Geometry check sheet. Reference: the model listing, model coordinates, mm. A direction names the side the tool comes from. Give positions to 0.01 mm unless a question says otherwise; leave off trailing zeros. Write each loop counter-clockwise with the first axis right and the second up, starting at its lowest first coordinate (ties: lowest second). Pieces come first, ordered by that corner, then holes.
(1) Cross-section at D-D (x = -11.5). Record the boundary of the cut face in (y, z) (3 decimals), and give its area (3 significant figures).
(2) Cross-section at C-C (z = 1.1). Count the separate pieces of the cut face and the enclosed holes in it, and give its area (3 significant figures).
(3) Thickness scan on line 1 along Y through (x, z) = (0, 2.65); line 2 along Y through (x, z) = (0, 3.95); line 3 along X through (y, z) = (-5.5, 0.45). Record the ranges inside material, lowest first.
(4) Tool access check on faces 3 (the flat face through (-11, -6.645, 2)), 4 (the cylindrical face through (-0.88, -3.94, 4.24)). Record the directions out of +Z, -Z, +X, -X, +Y, -Y that give a thin tool (end or side, any length) a straight path to the whole face; none if there is none.
(5) Mould release check, pull along X, two halves, no side actions. Record for faces 1 (the flat face through (6.645, -11, 2)), 2 (the flat face through (-5, 5, 0)): +X half, -X half, draft (parallel to the pull), parting line (faces both ways), or undercut.
(6) Depth check by flat-ended pin: P1, Ø1.4, axis at x = 12, y = -2.5, coming from the -Z side (3 decimals); P2, Ø0.7, axis at x = -11, z = 1, coming from the -Y side; P3, Ø1.2, axis at y = -10.5, z = 1, coming from the +X side. Enter the tip coordinate at first touch or a pass-through.
```python
from build123d import *

# Parameters (mm, degrees)
SKETCH1_R               = 15
BOSS_EXTRUDE1_DEPTH     = 5
CUT_EXTRUDE1_DEPTH      = 3.125
BOSS_EXTRUDE4_START     = 3.125
BOSS_EXTRUDE4_DEPTH     = 3.125
CIRPATTERN1_COUNT       = 4
SKETCH4_R               = 6
CUT_EXTRUDE2_DEPTH      = 3.5
FILLET1_R               = 0.25
CUT_EXTRUDE3_DEPTH      = 22.794494718
CUT_EXTRUDE3_DEPTH_BACK = 22.794494718
SKETCH5_R               = 4.0375
FILLET2_R               = 0.5


with BuildPart() as part:
    # Sketch1 → Boss-Extrude1 (new body)
    with BuildSketch(Plane.XY):
        Circle(SKETCH1_R)
    extrude(amount=BOSS_EXTRUDE1_DEPTH)

    # Sketch1_5 → Cut-Extrude1 (cut)
    with BuildSketch(Plane.XY):
        with BuildLine():
            ThreePointArc((-2.469224322, 13.9075), (-4.680749466, 13.326897968), (-6.769624128, 12.397088939))
            Line((-6.769624128, 12.397088939), (-6.769624128, 8.9075))
            Line((-6.769624128, 8.9075), (6.769624128, 8.9075))
            Line((6.769624128, 8.9075), (6.769624128, 12.397088939))
            ThreePointArc((6.769624128, 12.397088939), (4.680749466, 13.326897968), (2.469224322, 13.9075))
            Line((2.469224322, 13.9075), (-2.469224322, 13.9075))
        make_face()
    cut_extrude1 = extrude(amount=CUT_EXTRUDE1_DEPTH, mode=Mode.SUBTRACT)

    # Sketch7 → Boss-Extrude4 (add)
    with BuildSketch(Plane(origin=(0, 0, 3.125), x_dir=(-1, 0, 0), z_dir=(0, 0, -1)).offset(BOSS_EXTRUDE4_START)):
        with BuildLine():
            ThreePointArc((-2.469224322, 13.9075), (-4.680749466, 13.326897968), (-6.769624128, 12.397088939))
            Line((-6.769624128, 12.397088939), (-6.769624128, 8.9075))
            Line((-6.769624128, 8.9075), (6.769624128, 8.9075))
            Line((6.769624128, 8.9075), (6.769624128, 12.397088939))
            ThreePointArc((6.769624128, 12.397088939), (4.680749466, 13.326897968), (2.469224322, 13.9075))
            Line((2.469224322, 13.9075), (-2.469224322, 13.9075))
        make_face()
        with BuildLine():
            ThreePointArc((-2.45818912, 13.7825), (-4.609561284, 13.219377624), (-6.644624128, 12.322701416))
            Line((-6.644624128, 12.322701416), (-6.644624128, 9.0325))
            Line((-6.644624128, 9.0325), (6.644624128, 9.0325))
            Line((6.644624128, 9.0325), (6.644624128, 12.322701416))
            ThreePointArc((6.644624128, 12.322701416), (4.609561284, 13.219377624), (2.45818912, 13.7825))
            Line((2.45818912, 13.7825), (-2.45818912, 13.7825))
        make_face(mode=Mode.SUBTRACT)
    boss_extrude4 = extrude(amount=-BOSS_EXTRUDE4_DEPTH)

    # CirPattern1: Cut-Extrude1, Boss-Extrude4 ×4 about axis
    cirpattern1_axis = Axis((0, 0, 0), (0, 0, 1))
    add([cut_extrude1.rotate(cirpattern1_axis, i * 360 / CIRPATTERN1_COUNT) for i in range(1, CIRPATTERN1_COUNT)], mode=Mode.SUBTRACT)
    add([boss_extrude4.rotate(cirpattern1_axis, i * 360 / CIRPATTERN1_COUNT) for i in range(1, CIRPATTERN1_COUNT)])

    # Sketch4 → Cut-Extrude2 (cut)
    with BuildSketch(Plane(origin=(0, 0, 0), x_dir=(-1, 0, 0), z_dir=(0, 0, -1))):
        Circle(SKETCH4_R)
    extrude(amount=-CUT_EXTRUDE2_DEPTH, mode=Mode.SUBTRACT)

    # Fillet1
    fillet1_edges = [part.edges().sort_by_distance(p)[0] for p in [
        (6, 0, 0),
    ]]
    fillet(fillet1_edges, radius=FILLET1_R)

    # Sketch5 → Cut-Extrude3 (cut, two sides: drawn at the far end of the back side and taken through both)
    with BuildSketch(Plane.XY.offset(5).offset(-CUT_EXTRUDE3_DEPTH_BACK)):
        Circle(SKETCH5_R)
    extrude(amount=CUT_EXTRUDE3_DEPTH + CUT_EXTRUDE3_DEPTH_BACK, mode=Mode.SUBTRACT)

    # Fillet2
    fillet2_edges = [part.edges().sort_by_distance(p)[0] for p in [
        (-12.322701416, 6.644624128, 1.5625),
        (-13.7825, 2.45818912, 1.5625),
        (-13.7825, -2.45818912, 1.5625),
        (-12.322701416, -6.644624128, 1.5625),
        (-9.0325, -6.644624128, 1.5625),
        (-9.0325, 6.644624128, 1.5625),
        (-6.644624128, -12.322701416, 1.5625),
        (-2.45818912, -13.7825, 1.5625),
        (2.45818912, -13.7825, 1.5625),
        (6.644624128, -12.322701416, 1.5625),
        (6.644624128, -9.0325, 1.5625),
        (-6.644624128, -9.0325, 1.5625),
        (12.322701416, -6.644624128, 1.5625),
        (13.7825, -2.45818912, 1.5625),
        (13.7825, 2.45818912, 1.5625),
        (12.322701416, 6.644624128, 1.5625),
        (9.0325, 6.644624128, 1.5625),
        (9.0325, -6.644624128, 1.5625),
        (6.644624128, 12.322701416, 1.5625),
        (2.45818912, 13.7825, 1.5625),
        (-2.45818912, 13.7825, 1.5625),
        (-6.644624128, 12.322701416, 1.5625),
        (-6.644624128, 9.0325, 1.5625),
        (6.644624128, 9.0325, 1.5625),
    ]]
    fillet(fillet2_edges, radius=FILLET2_R)


solid = part.part
```
Reply:
1. outline: (-9.631, 0) - (-6.645, 0) - (-6.645, 3.125) - (6.645, 3.125) - (6.645, 0) - (9.631, 0) - (9.631, 5) - (-9.631, 5) - close
1. area: 54.8 mm2
2. separate pieces: 1
2. enclosed holes: 5
2. area: 362 mm2
3. line 1: y = -15 to -13.78, -9.03 to -6, 6 to 9.03, 13.78 to 15
3. line 2: y = -15 to -4.04, 4.04 to 15
3. line 3: x = -13.96 to -12.87, -9.03 to -2.4, 2.4 to 9.03, 12.87 to 13.96
4. face 3: -Z
4. face 4: +Z, -Z
5. face 1: undercut
5. face 2: draft
6. P1: stops at z = 3.125
6. P2: stops at y = -10.56
6. P3: stops at x = 11.27
